from build123d import *

# Parameters (mm, degrees)
SKETCH1_R           = 5
BOSS_EXTRUDE1_DEPTH = 125


with BuildPart() as part:
    # Sketch1 → Boss-Extrude1 (new body, symmetric)
    with BuildSketch(Plane(origin=(0, 0, 0), x_dir=(0, 0, -1), z_dir=(1, 0, 0))):
        Circle(SKETCH1_R)
    extrude(amount=BOSS_EXTRUDE1_DEPTH, both=True)

    # Sketch2 → Revolve1 (revolve)
    with BuildSketch(Plane(origin=(125, 0, 0), x_dir=(0, 0, -1), z_dir=(1, 0, 0))):
        with BuildLine():
            Line((0, 10), (0, -10))
            ThreePointArc((0, -10), (10, 0), (0, 10))
        make_face()
    revolve1 = revolve(axis=Axis((125, 10, 0), (0, -1, 0)))

    # Mirror1: Revolve1 across plane
    add(revolve1.mirror(Plane(origin=(0, 0, 0), x_dir=(0, 0, 1), z_dir=(1, 0, 0))))


solid = part.part
Design review of the part built by this model. Coordinates are the model's own, in mm. Give positions to 0.01 mm unless a question says otherwise; leave off trailing zeros. Loops run counter-clockwise (first coordinate to the right, second up) from the corner with the lowest first, then second, coordinate; pieces in that order, holes last. Notation, with made-up numbers: (27, 71.5) - (57, 71.5) arc R21 cw to (57, 100.5) - close; hole circle Ø5 at (-35, -8.75). An arc over 180 degrees is marked (long way). Write item = value, one per line.
1) To check wall thickness, follow line 1 (X direction, y = 0, z = 5.5); line 2 (X direction, y = 6, z = 7); line 3 (Y direction, x = -63.5, z = -1.25). State the ranges of each line that lie inside material, in increasing order.
Result sheet:
line_1 = -133.35 to -116.65, 116.65 to 133.35
line_2 = -128.87 to -121.13, 121.13 to 128.87
line_3 = -4.84 to 4.84
2) Clearance check with flat-ended pins moving along their axes: pin 1 Ø12 at (y, z) = (6.5, 3.5) entering from -X; pin 2 Ø5 at (x, z) = (-64, 3.5) entering from -Y; pin 3 Ø2 at (y, z) = (-3, -7) entering from +X. State where each tip first meets the part, or that it passes through.
Result sheet:
pin_1 = -134.9
pin_2 = -4.9
pin_3 = 132.5
3) Take a section at A-A on y = 0. State the section outline as (x, z) points, and give its area (3 significant figures).
Result sheet:
outline = (-116.34, -5) - (116.34, -5) arc R10 ccw (long way) to (116.34, 5) - (-116.34, 5) arc R10 ccw (long way) to start
area = 2,940 mm2
4) Take a section at B-B on x = 56. State the section outline as (y, z) points.
Result sheet:
outline = circle Ø10 at (0, 0)
